Part print with two shaded views. Sizes in mm from the minimum x, y, z corner. A direction names the side the tool comes from. Coordinates: 2 decimals unless noted, no trailing zeros. Loops run counter-clockwise (first coordinate to the right, second up) from the corner with the lowest first, then second, coordinate; pieces in that order, holes last. Notation, with made-up numbers: (19, 78) -> (58, 78) arc R28 ccw to (58, 102) -> close; hole circle Ø4 at (4.25, 42.5). An arc over 180 degrees is marked (long way). Write each question's results on one line, items separated by ' | '.
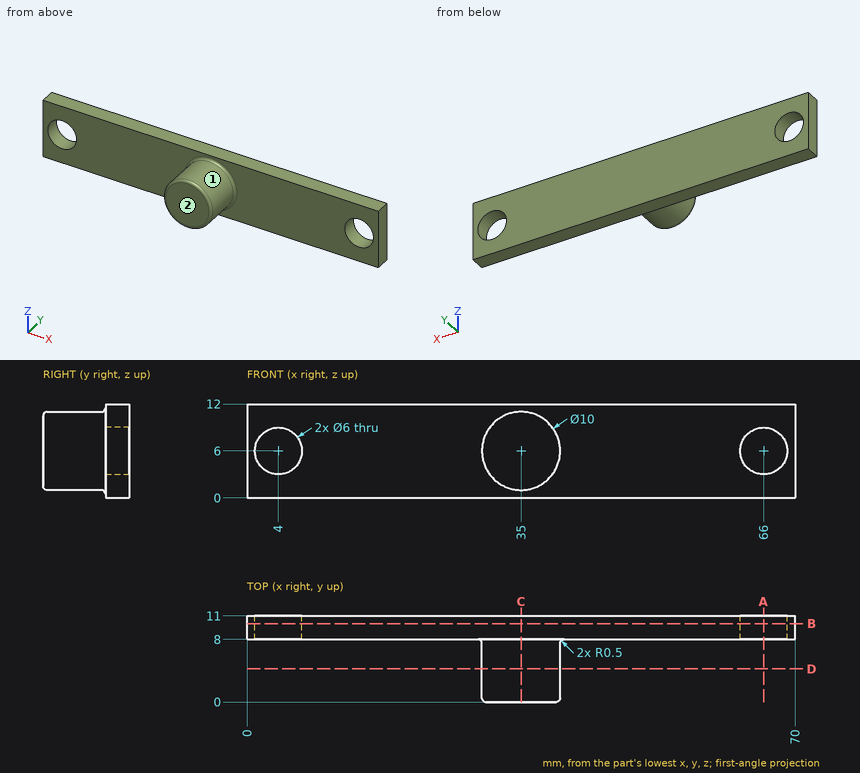
Q1. Cut at D-D on y = 4.25. Write the cut outline in (x, z), and give its area (3 significant figures).
Results are:
outline: circle Ø10 at (35, 6) | area: 78.5 mm^2
Q2. Drop flat-ended pins along their axis: pin 1 (6 mm diameter, centred on x = 25, z = 4, fed in from -Y); pin 2 (3 mm diameter, centred on y = 2, z = 5.5, fed in from -X). Give the stop position or say it passes through.
Results are:
pin 1: y = 8 | pin 2: x = 30
Q3. Cut at C-C on x = 35. Write the cut outline in (y, z).
Results are:
outline: (0, 1.5) arc R0.5 ccw to (0.5, 1) -> (7.5, 1) arc R0.5 cw to (8, 0.5) -> (8, 0) -> (11, 0) -> (11, 12) -> (8, 12) -> (8, 11.5) arc R0.5 cw to (7.5, 11) -> (0.5, 11) arc R0.5 ccw to (0, 10.5) -> close
Q4. Which spindle directions (+Z, -Z, +X, -X, +Y, -Y) get a long thin tool onto all of the face, cutting with end or side? Do the marked faces 1 and 2. Say none if no direction does.
Results are:
face 1: -Y | face 2: +Z, -Z, +X, -X, -Y
Q5. Cut at B-B on y = 10. Write the cut outline in (x, z), and give its area (3 significant figures).
Results are:
outline: (0, 0) -> (70, 0) -> (70, 12) -> (0, 12) -> close; hole circle Ø6 at (4, 6); hole circle Ø6 at (66, 6) | area: 783 mm^2
Q6. Cut at A-A on x = 66. Write the cut outline in (y, z), and give its area (3 significant figures).
Results are:
outline: (8, 0) -> (11, 0) -> (11, 3) -> (8, 3) -> close; (8, 9) -> (11, 9) -> (11, 12) -> (8, 12) -> close | area: 18.0 mm^2
Q7. Wall check: L1, parallel to X at y = 8.85, z = 6; L2, parallel to Y at x = 7.5, z = 2.5; L3, parallel to Z at x = 37, y = 3.75. Give the ranges that are in metal, low to high. Write a range as from..to.
Results are:
L1: 0..1, 7..63, 69..70 | L2: 8..11 | L3: 1.42..10.58
